from build123d import *

# Parameters (mm, degrees)
SKETCH_W        = 150
SKETCH_H        = 110
PAD_DEPTH       = 1.5875
SKETCH001_R     = 1.5
SKETCH001_R_2   = 12
SKETCH001_R_3   = 2
SKETCH001_W     = 58.5
SKETCH001_H     = 40
POCKET_DEPTH    = 1.5885
SKETCH002_R     = 1.5
SKETCH002_W     = 38.5
SKETCH002_H     = 8
SKETCH002_W_2   = 14
SKETCH002_H_2   = 13.5
SKETCH002_W_3   = 17
POCKET001_DEPTH = 1.5885
SKETCH003_R     = 2.5
SKETCH003_R_2   = 1.5
PAD001_DEPTH    = 6.35
POCKET002_DEPTH = 1.5885
FILLET_R        = 10


with BuildPart() as part:
    # Sketch → Pad (new body)
    with BuildSketch(Plane.XZ):
        with Locations((20, -10)):
            Rectangle(SKETCH_W, SKETCH_H)
    extrude(amount=PAD_DEPTH)

    # Sketch001 (on Face5 of Pad) → Pocket (cut, through all)
    with BuildSketch(Plane(origin=(0, 0, 0), x_dir=(1, 0, 0), z_dir=(0, 1, 0))):
        with Locations((-26.5, 5.07)):
            Circle(SKETCH001_R)
        with Locations((-26.5, -35.07)):
            Circle(SKETCH001_R)
        with Locations((66.5, -35.07)):
            Circle(SKETCH001_R)
        with Locations((66.5, 5.07)):
            Circle(SKETCH001_R)
        with Locations((-16.97, -18.72)):
            Circle(SKETCH001_R_2)
        with Locations((-16.97, -0.68)):
            Circle(SKETCH001_R_3)
        with Locations((34.15, -15)):
            Rectangle(SKETCH001_W, SKETCH001_H)
    extrude(amount=-POCKET_DEPTH, mode=Mode.SUBTRACT)

    # Sketch002 (on Face4 of Pocket) → Pocket001 (cut, through all)
    with BuildSketch(Plane(origin=(0, 0, 0), x_dir=(1, 0, 0), z_dir=(0, 1, 0))):
        with Locations((36.45, 25)):
            Circle(SKETCH002_R)
        with Locations((83.55, 25)):
            Circle(SKETCH002_R)
        with Locations((-38.6, 25)):
            Circle(SKETCH002_R)
        with Locations((-13.5, 25)):
            Circle(SKETCH002_R)
        with Locations((60, 25)):
            Rectangle(SKETCH002_W, SKETCH002_H)
        with Locations((11.5, 25)):
            Rectangle(SKETCH002_W_2, SKETCH002_H_2)
        with Locations((-26.05, 25)):
            Rectangle(SKETCH002_W_3, SKETCH002_H)
    extrude(amount=-POCKET001_DEPTH, mode=Mode.SUBTRACT)

    # Sketch003 (on Face4 of Pocket001) → Pad001 (join)
    with BuildSketch(Plane(origin=(0, 0, 0), x_dir=(1, 0, 0), z_dir=(0, 1, 0))):
        with Locations((-26.5, 5.07)):
            Circle(SKETCH003_R)
        with Locations((-26.5, 5.07)):
            Circle(SKETCH003_R_2, mode=Mode.SUBTRACT)
        with Locations((-26.5, -35.07)):
            Circle(SKETCH003_R)
        with Locations((-26.5, -35.07)):
            Circle(SKETCH003_R_2, mode=Mode.SUBTRACT)
        with Locations((66.5, 5.07)):
            Circle(SKETCH003_R)
        with Locations((66.5, 5.07)):
            Circle(SKETCH003_R_2, mode=Mode.SUBTRACT)
        with Locations((66.5, -35.07)):
            Circle(SKETCH003_R)
        with Locations((66.5, -35.07)):
            Circle(SKETCH003_R_2, mode=Mode.SUBTRACT)
    extrude(amount=-PAD001_DEPTH)

    # Sketch004 (on Face5 of Pad001) → Pocket002 (cut, through all)
    with BuildSketch(Plane.XZ.offset(1.5875)):
        with BuildLine():
            ThreePointArc((-26.17718, -38.575536), (-34.73218, -47.130536), (-26.17718, -55.685536))
            Line((-26.17718, -55.685536), (70.560877, -55.685536))
            ThreePointArc((70.560877, -55.685536), (79.115877, -47.130536), (70.560877, -38.575536))
            Line((-26.17718, -38.575536), (70.560877, -38.575536))
        make_face()
        with BuildLine():
            ThreePointArc((-33.215195, 29.997324), (-41.77, 38.552129), (-50.324805, 29.997324))
            Line((-50.324805, 29.997324), (-50.324805, -4.910724))
            ThreePointArc((-50.324805, -4.910724), (-41.77, -13.465529), (-33.215195, -4.910724))
            Line((-33.215195, 29.997324), (-33.215195, -4.910724))
        make_face()
        with BuildLine():
            ThreePointArc((89.482501, 29.997324), (81.764, 37.715825), (74.045499, 29.997324))
            Line((74.045499, 29.997324), (74.045499, -4.910724))
            ThreePointArc((74.045499, -4.910724), (81.764, -12.629225), (89.482501, -4.910724))
            Line((89.482501, 29.997324), (89.482501, -4.910724))
        make_face()
    extrude(amount=-POCKET002_DEPTH, mode=Mode.SUBTRACT)

    # Fillet
    fillet_edges = [part.edges().sort_by_distance(p)[0] for p in [
        (95, -0.79375, 45),
        (-55, -0.79375, 45),
    ]]
    fillet(fillet_edges, radius=FILLET_R)


solid = part.part
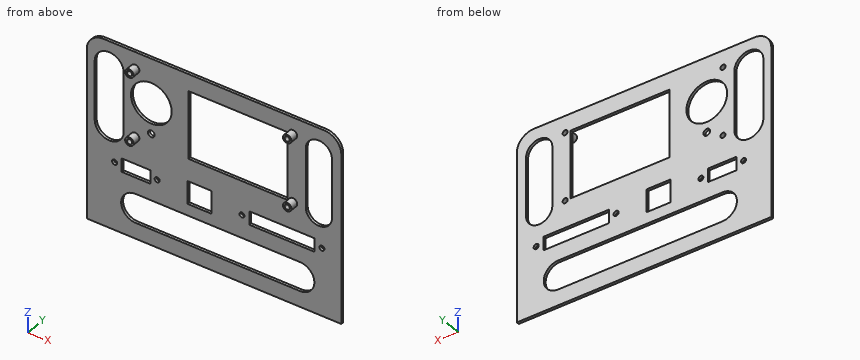
Build history of the part. All positions in model axes, mm. Coordinates: 2 decimals unless noted, no trailing zeros. Order: outer loops, then holes, each group sorted by start corner. A loop starts at its lowest first (then second) coordinate and runs counter-clockwise, first axis right, second up. Notation, with made-up numbers: (35, 75.25) - (70, 75.25) arc R32 ccw to (70, 102.25) - close; hole circle Ø10 at (-2.5, 63). An arc over 180 degrees is marked (long way). Write each question's results on one line, items separated by ' | '. Start each with the question number.
Item 1: Band-saw the part on B-B on z = 0.68. Write the cut outline in (x, y).
Item 2: Flat gauge pins, fed straight in: pin 1 (2 mm diameter, centred on x = -10.5, y = -4, fed in from +Z); pin 2 (5 mm diameter, centred on x = -26.5, z = 35.07, fed in from -Y). Where does each tip first touch, or does it go through?
Item 3: Band-saw the part on C-C on x = -41.77. Write the cut outline in (y, z), and give its area (3 significant figures).
Item 4: Band-saw the part on D-D on z = 18.72. Write the cut outline in (x, y).
Item 5: Band-saw the part on A-A on x = 13.5. Write the cut outline in (y, z), and give its area (3 significant figures).
Item 6: Wall check: probe 1 along Z at (x, y) = (-16.97, -0.6); probe 2 along Z at (x, y) = (66.5, -1.25); probe 3 along X at (y, z) = (-1.5, -5.07). Give the ranges that are in metal, low to high. Write a range as [from, to].
Numbers:
1) outline: (-55, -1.59) - (-50.32, -1.59) - (-50.32, 0) - (-55, 0) - close; (-33.22, -1.59) - (-18.97, -1.59) - (-18.97, 0) - (-33.22, 0) - close; (-14.97, -1.59) - (4.9, -1.59) - (4.9, 0) - (-14.97, 0) - close; (63.4, -1.59) - (74.05, -1.59) - (74.05, 0) - (63.4, 0) - close; (89.48, -1.59) - (95, -1.59) - (95, 0) - (89.48, 0) - close
2) pin 1: through | pin 2: y = -6.35
3) outline: (-1.59, -65) - (0, -65) - (0, -13.47) - (-1.59, -13.47) - close; (-1.59, 38.55) - (0, 38.55) - (0, 45) - (-1.59, 45) - close | area: 92.0 mm^2
4) outline: (-55, -1.59) - (-50.32, -1.59) - (-50.32, 0) - (-55, 0) - close; (-33.22, -1.59) - (-28.97, -1.59) - (-28.97, 0) - (-33.22, 0) - close; (-4.97, -1.59) - (4.9, -1.59) - (4.9, 0) - (-4.97, 0) - close; (63.4, -1.59) - (74.05, -1.59) - (74.05, 0) - (63.4, 0) - close; (89.48, -1.59) - (95, -1.59) - (95, 0) - (89.48, 0) - close
5) outline: (-1.59, -65) - (0, -65) - (0, -55.69) - (-1.59, -55.69) - close; (-1.59, -38.58) - (0, -38.58) - (0, -31.75) - (-1.59, -31.75) - close; (-1.59, -18.25) - (0, -18.25) - (0, -5) - (-1.59, -5) - close; (-1.59, 35) - (0, 35) - (0, 45) - (-1.59, 45) - close | area: 62.5 mm^2
6) probe 1: [-65, -55.69], [-38.58, -1.32], [2.68, 6.72], [30.72, 45] | probe 2: [-65, -55.69], [-38.58, -29], [-21, -6.57], [-3.57, 33.57], [36.57, 45] | probe 3: [-55, -50.32], [-33.22, -28], [-25, 65], [68, 74.05], [89.48, 95]
